```python
from build123d import *

# Parameters (mm, degrees)
BOSS_EXTRUDE1_DEPTH  = 32
SKETCH5_R            = 16
SKETCH5_R_2          = 8
BOSS_EXTRUDE2_DEPTH  = 22
CUT_EXTRUDE1_REACH   = 146
SKETCH9_R            = 3
CUT_EXTRUDE2_DEPTH   = 10
LPATTERN1_COUNT      = 2
LPATTERN1_PITCH      = 70
LPATTERN1_COUNT_DIR2 = 2
LPATTERN1_PITCH_DIR2 = 44


with BuildPart() as part:
    # Sketch3 → Boss-Extrude1 (new body, symmetric)
    with BuildSketch(Plane.XY):
        Polygon((0, 0), (0, 42.452913403), (12.839514692, 52), (22.839514692, 52), (22.839514692, 16), (144, 16), (144, 0), align=None)
    extrude(amount=BOSS_EXTRUDE1_DEPTH, both=True)

    # Sketch5 → Boss-Extrude2 (add)
    with BuildSketch(Plane(origin=(144, 0, 0), x_dir=(0, 0, -1), z_dir=(1, 0, 0))):
        with Locations((0, 36)):
            Circle(SKETCH5_R)
        with Locations((0, 36)):
            Circle(SKETCH5_R_2, mode=Mode.SUBTRACT)
        with BuildLine():
            ThreePointArc((16, 36), (-3.463033823, 20.379263886), (-14.500924593, 42.761892188))
            Line((-14.500924593, 42.761892188), (-26.172487288, 17.732145215))
            ThreePointArc((-26.172487288, 17.732145215), (-27.279511824, 16.469825663), (-28.891410649, 16))
            Line((-28.891410649, 16), (28.891410649, 16))
            ThreePointArc((28.891410649, 16), (27.279511824, 16.469825663), (26.172487288, 17.732145215))
            Line((26.172487288, 17.732145215), (14.500924593, 42.761892188))
            ThreePointArc((14.500924593, 42.761892188), (15.620736114, 39.463033823), (16, 36))
        make_face()
    extrude(amount=-BOSS_EXTRUDE2_DEPTH)

    # Sketch8 → Cut-Extrude1 (cut, up to next)
    with BuildSketch(Plane(origin=(144, 0, 0), x_dir=(0, 0, -1), z_dir=(1, 0, 0)), mode=Mode.PRIVATE) as cut_extrude1_sk1:
        Polygon((-16, 0), (-16, 7), (-8, 7), (-8, 16), (8, 16), (8, 7), (16, 7), (16, 0), align=None)
    cut_extrude1_tool1 = extrude(cut_extrude1_sk1.sketch, amount=-CUT_EXTRUDE1_REACH, mode=Mode.PRIVATE) & part.part
    add(cut_extrude1_tool1.solids().sort_by_distance((144, 6.630435, 0))[0], mode=Mode.SUBTRACT)

    # Sketch9 → Cut-Extrude2 (cut)
    with BuildSketch(Plane.XZ):
        with Locations((38, 22)):
            Circle(SKETCH9_R)
    cut_extrude2 = extrude(amount=-CUT_EXTRUDE2_DEPTH, mode=Mode.SUBTRACT)

    # LPattern1: Cut-Extrude2 2 × 2
    with Locations(*[(i * LPATTERN1_PITCH, 0, -j * LPATTERN1_PITCH_DIR2) for i in range(LPATTERN1_COUNT) for j in range(LPATTERN1_COUNT_DIR2) if (i, j) != (0, 0)]):
        add(cut_extrude2, mode=Mode.SUBTRACT)


solid = part.part
```
Read the model definition and answer for the solid it produces. Units are mm, in the model's axes. A direction names the side the tool comes from. Round coordinates to 2 decimals unless told otherwise and drop trailing zeros. Write each loop counter-clockwise with the first axis right and the second up, starting at its lowest first coordinate (ties: lowest second). Pieces come first, ordered by that corner, then holes. Notation, with made-up numbers: (-27.5, 35) -> (9.5, 35) arc R23 cw to (9.5, 57) -> close; hole circle Ø9 at (52.5, -18.5). An arc over 180 degrees is marked (long way). Answer in a Markdown table with one row per item. Add a question column.
1) Find section C-C, the plane z = 5. Determine the outline of the cut face in (x, y) (3 decimals), and give its area (3 significant figures).
2) Given P1, Ø18, axis at y = 34.5, z = 3.5, coming from the +X side; P2, Ø19, axis at x = 81, z = -21, coming from the +Y side; P3, Ø3.5, axis at x = 108, z = -22, coming from the -Y side; P4, Ø1, axis at x = 42.5, z = 10.5, coming from the -Y side, each flat-ended and moving along its own axis, determine where each tip first touches the part or whether it passes through.
3) Find section B-B, the plane x = 90. Determine the outline of the cut face in (y, z).
4) Consider line 1 (Z direction, x = 108, y = 7.5); line 2 (Z direction, x = 108, y = 6.5); line 3 (Z direction, x = 77.5, y = 6). Determine where each line is inside the solid, lowest interval first.
5) Find section D-D, the plane z = -10. Determine the outline of the cut face in (x, y).
6) Determine the mould class of faces 1 (the face through (73, 7, -12)), 2 (the face through (35, 5, 22)) for opening direction X: pulls with the +X half, pulls with the -X half, needs draft (parallel to the pull), parting line crosses it, or undercut.
7) Which of the six approach directions +Z, -Z, +X, -X, +Y, -Y give full straight-line access (tool end or side, diameter ignored) to faces 3 (the face through (22.84, 34, 0)), 4 (the face through (110.86, 4.93, 22.9)), 5 (the face through (133.154, 30.422, 20.255)), 6 (the face through (73, 7, 12))?
8) Find section A-A, the plane y = 5. Determine the outline of the cut face in (x, z), and give its area (3 significant figures).
Findings below:
| question | item | result |
|---|---|---|
| 1 | outline | (0, 16) -> (22.84, 16) -> (22.84, 52) -> (12.84, 52) -> (0, 42.453) -> close; (122, 16) -> (144, 16) -> (144, 29.755) -> (122, 29.755) -> close; (122, 42.245) -> (144, 42.245) -> (144, 51.199) -> (122, 51.199) -> close |
| 1 | area | 1,260 mm² |
| 2 | P1 | x = 144 |
| 2 | P2 | y = 16 |
| 2 | P3 | y = 10 |
| 2 | P4 | y = 7 |
| 3 | outline | (0, -32) -> (16, -32) -> (16, -8) -> (7, -8) -> (7, -16) -> (0, -16) -> close; (0, 16) -> (7, 16) -> (7, 8) -> (16, 8) -> (16, 32) -> (0, 32) -> close |
| 4 | line 1 | -32 to -25, -19 to -8, 8 to 19, 25 to 32 |
| 4 | line 2 | -32 to -25, -19 to -16, 16 to 19, 25 to 32 |
| 4 | line 3 | -32 to -16, 16 to 32 |
| 5 | outline | (0, 7) -> (144, 7) -> (144, 48.49) -> (122, 48.49) -> (122, 16) -> (22.84, 16) -> (22.84, 52) -> (12.84, 52) -> (0, 42.45) -> close |
| 6 | face 1 | needs draft |
| 6 | face 2 | undercut |
| 7 | face 3 | +Z, -Z, +Y |
| 7 | face 4 | -Y |
| 7 | face 5 | +Z, +X, +Y |
| 7 | face 6 | +X, -X, -Y |
| 8 | outline | (0, -32) -> (144, -32) -> (144, -16) -> (0, -16) -> close; (0, 16) -> (144, 16) -> (144, 32) -> (0, 32) -> close; hole circle Ø6 at (38, -22); hole circle Ø6 at (38, 22); hole circle Ø6 at (108, -22); hole circle Ø6 at (108, 22) |
| 8 | area | 4,490 mm² |
